Geometry check sheet. Reference: the model listing, model coordinates, mm. Face numbers are marked on the shaded views. A direction names the side the tool comes from. Give positions to 0.01 mm unless a question says otherwise; leave off trailing zeros. Write each loop counter-clockwise with the first axis right and the second up, starting at its lowest first coordinate (ties: lowest second). Pieces come first, ordered by that corner, then holes. Notation, with made-up numbers: (-18, 50.25) - (-12, 50.25) arc R28 ccw to (-12, 81.25) - close; hole circle Ø2 at (-39, -34.5). An arc over 180 degrees is marked (long way). One line per question, with ' | ' between items. Start each with the question number.
Q1. Thickness scan on L1, parallel to X at y = 51, z = 0; L2, parallel to Y at x = -13.5, z = 12; L3, parallel to X at y = 66.5, z = -15.5. Record the ranges inside material, lowest first. Write a range as [from, to].
Q2. Gauge pin test, flat ends, axial feed: P1, Ø4, axis at x = -10, y = 40, coming from the -Z side; P2, Ø5, axis at y = 67, z = -1.5, coming from the -X side; P3, Ø11, axis at y = 67.5, z = -0.5, coming from the +X side. Record the tip position at first contact, or that the pin passes through.
Q3. Section check D-D on z = 14. Record the boundary of the cut face in (x, y), and give its area (3 significant figures).
Q4. Section check B-B on y = 7. Record the boundary of the cut face in (x, z), and give its area (3 significant figures).
Q5. Set-up check for the marked faces 5, 6, 7, 8 and 9: record each of +Z, -Z, +X, -X, +Y, -Y from which the full face is reachable in a straight line by a thin tool's end or side.
Q6. Section check A-A on x = 0. Record the boundary of the cut face in (y, z).
Q7. Section check C-C on z = -8.5. Record the boundary of the cut face in (x, y).
Q8. Release check for a two-part mould opening along Y. For the marked faces 1, 2, 3 and 4 record: +Y half, -Y half, draft (parallel to the pull), parting line (faces both ways), or undercut.
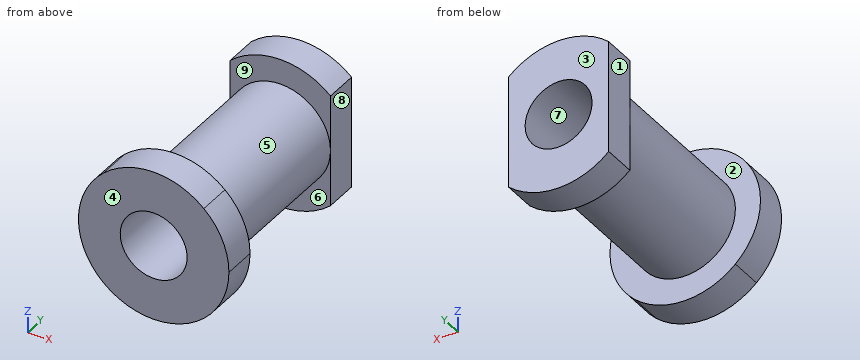
```python
from build123d import *

# Parameters (mm, degrees)
BOSS_EXTRUDE1_DEPTH = 10
SKETCH1_3_R         = 15
SKETCH1_3_R_2       = 10
BOSS_EXTRUDE2_DEPTH = 70
BOSS_EXTRUDE3_START = 60
BOSS_EXTRUDE3_DEPTH = 10


with BuildPart() as part:
    # Sketch1 → Boss-Extrude1 (new body)
    with BuildSketch(Plane(origin=(0, 0, 0), x_dir=(1, 0, 0), z_dir=(0, 1, 0))):
        with BuildLine():
            Line((15, 0), (15, -16.770509831))
            ThreePointArc((15, -16.770509831), (20.539595906, -9.185586535), (22.5, 0))
            ThreePointArc((22.5, 0), (20.539595906, 9.185586535), (15, 16.770509831))
            Line((15, 16.770509831), (15, 0))
        make_face()
        with BuildLine():
            ThreePointArc((-15, -16.770509831), (0, -22.5), (15, -16.770509831))
            Line((15, -16.770509831), (15, 0))
            ThreePointArc((15, 0), (-7e-09, -15), (-15, 1.4e-08))
            Line((-15, 1.4e-08), (-15, -16.770509831))
        make_face()
        with BuildLine():
            ThreePointArc((-15, 1.4e-08), (7e-09, 15), (15, 0))
            Line((15, 0), (15, 16.770509831))
            ThreePointArc((15, 16.770509831), (0, 22.5), (-15, 16.770509831))
            Line((-15, 16.770509831), (-15, 1.4e-08))
        make_face()
        with BuildLine():
            ThreePointArc((-15, 16.770509831), (-22.5, 0), (-15, -16.770509831))
            Line((-15, -16.770509831), (-15, 1.4e-08))
            Line((-15, 1.4e-08), (-15, 16.770509831))
        make_face()
    extrude(amount=BOSS_EXTRUDE1_DEPTH)

    # Sketch1_3 → Boss-Extrude2 (add)
    with BuildSketch(Plane(origin=(0, 0, 0), x_dir=(1, 0, 0), z_dir=(0, 1, 0))):
        with Locations(Location((0, 0, 0), (0, 0, 270))):
            Circle(SKETCH1_3_R)
        with Locations(Location((0, 0, 0), (0, 0, 270))):
            Circle(SKETCH1_3_R_2, mode=Mode.SUBTRACT)
    extrude(amount=BOSS_EXTRUDE2_DEPTH)

    # Sketch1_4 → Boss-Extrude3 (add)
    with BuildSketch(Plane(origin=(0, 0, 0), x_dir=(1, 0, 0), z_dir=(0, 1, 0)).offset(BOSS_EXTRUDE3_START)):
        with BuildLine():
            ThreePointArc((-15, -16.770509831), (0, -22.5), (15, -16.770509831))
            Line((15, -16.770509831), (15, 0))
            ThreePointArc((15, 0), (-7e-09, -15), (-15, 1.4e-08))
            Line((-15, 1.4e-08), (-15, -16.770509831))
        make_face()
        with BuildLine():
            ThreePointArc((-15, 1.4e-08), (7e-09, 15), (15, 0))
            Line((15, 0), (15, 16.770509831))
            ThreePointArc((15, 16.770509831), (0, 22.5), (-15, 16.770509831))
            Line((-15, 16.770509831), (-15, 1.4e-08))
        make_face()
    extrude(amount=BOSS_EXTRUDE3_DEPTH)


solid = part.part
```
Working result:
1) L1: x = [-15, -10], [10, 15] | L2: y = [0, 10], [60, 70] | L3: x = [-15, 15]
2) P1: stops at z = -12.69 | P2: stops at x = -15 | P3: stops at x = 15
3) outline: (-17.61, 0) - (17.61, 0) - (17.61, 10) - (5.39, 10) - (5.39, 60) - (15, 60) - (15, 70) - (-15, 70) - (-15, 60) - (-5.39, 60) - (-5.39, 10) - (-17.61, 10) - close | area: 1,190 mm2
4) outline: circle Ø45 at (0, 0); hole circle Ø20 at (0, 0) | area: 1,280 mm2
5) face 5: none | face 6: -Z | face 7: +Y, -Y | face 8: +Z, -Z, +X, +Y | face 9: +Z
6) outline: (0, -22.5) - (10, -22.5) - (10, -15) - (60, -15) - (60, -22.5) - (70, -22.5) - (70, -10) - (0, -10) - close; (0, 10) - (70, 10) - (70, 22.5) - (60, 22.5) - (60, 15) - (10, 15) - (10, 22.5) - (0, 22.5) - close
7) outline: (-20.83, 0) - (-5.27, 0) - (-5.27, 70) - (-15, 70) - (-15, 60) - (-12.36, 60) - (-12.36, 10) - (-20.83, 10) - close; (5.27, 0) - (20.83, 0) - (20.83, 10) - (12.36, 10) - (12.36, 60) - (15, 60) - (15, 70) - (5.27, 70) - close
8) face 1: draft | face 2: undercut | face 3: +Y half | face 4: -Y half
